from build123d import *

# Parameters (mm, degrees)
BOSS_EXTRUDE1_DEPTH = 3
SKETCH2_R           = 1.25
CUT_EXTRUDE1_DEPTH  = 16
CHAMFER1_SIZE       = 0.25
SKETCH3_R           = 4
CUT_EXTRUDE2_DEPTH  = 1
CUT_EXTRUDE3_DEPTH  = 11
CUT_EXTRUDE4_DEPTH  = 2
FILLET1_R           = 0.25
CUT_EXTRUDE5_DEPTH  = 3
SKETCH7_R           = 2.35
CUT_EXTRUDE6_DEPTH  = 3.5
CUT_EXTRUDE7_DEPTH  = 3.5
CIRPATTERN1_COUNT   = 24


with BuildPart() as part:
    # Sketch1 → Boss-Extrude1 (new body, symmetric)
    with BuildSketch(Plane(origin=(0, 0, 0), x_dir=(1, 0, 0), z_dir=(0, 1, 0))):
        with BuildLine():
            Line((23.75, 3.122009569), (9.501734608, 3.122009569))
            ThreePointArc((9.501734608, 3.122009569), (7.409369814, 3.580863286), (5.701040765, 4.873205742))
            ThreePointArc((5.701040765, 4.873205742), (-7.499303275, 0.102227183), (5.566088347, -5.026794258))
            ThreePointArc((5.566088347, -5.026794258), (7.246540637, -3.808746464), (9.276813911, -3.377990431))
            Line((9.276813911, -3.377990431), (23.75, -3.377990431))
            ThreePointArc((23.75, -3.377990431), (27, -0.127990431), (23.75, 3.122009569))
        make_face()
    extrude(amount=BOSS_EXTRUDE1_DEPTH, both=True)

    # Sketch2 → Cut-Extrude1 (cut)
    with BuildSketch(Plane(origin=(0, 3, 0), x_dir=(1, 0, 0), z_dir=(0, 1, 0))):
        with Locations((23.75, -0.127990431)):
            Circle(SKETCH2_R)
        with Locations((19.75, -0.127990431)):
            Circle(SKETCH2_R)
    extrude(amount=-CUT_EXTRUDE1_DEPTH, mode=Mode.SUBTRACT)

    # Chamfer1
    chamfer1_edges = [part.edges().sort_by_distance(p)[0] for p in [
        (22.5, 3, 0.127990431),
        (18.5, 3, 0.127990431),
    ]]
    chamfer(chamfer1_edges, length=CHAMFER1_SIZE)

    # Sketch3 → Cut-Extrude2 (cut)
    with BuildSketch(Plane(origin=(0, 3, 0), x_dir=(1, 0, 0), z_dir=(0, 1, 0))):
        Circle(SKETCH3_R)
    extrude(amount=-CUT_EXTRUDE2_DEPTH, mode=Mode.SUBTRACT)

    # Sketch4 → Cut-Extrude3 (cut)
    with BuildSketch(Plane(origin=(0, 3, 0), x_dir=(1, 0, 0), z_dir=(0, 1, 0))):
        with BuildLine():
            Line((-1.5, 1), (-9, 1))
            Line((-9, 1), (-9, -1))
            Line((-9, -1), (-1.5, -1))
            ThreePointArc((-1.5, -1), (-1.183772234, -1.051316702), (-0.9, -1.2))
            ThreePointArc((-0.9, -1.2), (0, -1.5), (0.9, -1.2))
            ThreePointArc((0.9, -1.2), (1.183772234, -1.051316702), (1.5, -1))
            Line((1.5, -1), (7.969223594, -1))
            ThreePointArc((7.969223594, -1), (8.204925854, -1.028174684), (8.427346441, -1.111111111))
            ThreePointArc((8.427346441, -1.111111111), (10.25, 0), (8.427346441, 1.111111111))
            ThreePointArc((8.427346441, 1.111111111), (8.204925854, 1.028174684), (7.969223594, 1))
            Line((7.969223594, 1), (1.5, 1))
            ThreePointArc((1.5, 1), (1.183772234, 1.051316702), (0.9, 1.2))
            ThreePointArc((0.9, 1.2), (0, 1.5), (-0.9, 1.2))
            ThreePointArc((-0.9, 1.2), (-1.183772234, 1.051316702), (-1.5, 1))
        make_face()
    extrude(amount=-CUT_EXTRUDE3_DEPTH, mode=Mode.SUBTRACT)

    # Sketch5 → Cut-Extrude4 (cut)
    with BuildSketch(Plane.XZ.offset(3)):
        with BuildLine():
            Line((24.055684797, -4.372009569), (19.49, -4.372009569))
            Line((19.49, -4.372009569), (6.737511188, -4.372009569))
            ThreePointArc((6.737511188, -4.372009569), (8.030233116, 0.154534121), (6.564314835, 4.627990431))
            Line((6.564314835, 4.627990431), (19.49, 4.627990431))
            Line((19.49, 4.627990431), (24.055684797, 4.627990431))
            ThreePointArc((24.055684797, 4.627990431), (27.230594245, 3.312899878), (28.545684797, 0.137990431))
            Line((28.545684797, 0.137990431), (28.545684797, 0.117990431))
            ThreePointArc((28.545684797, 0.117990431), (27.230594245, -3.056919017), (24.055684797, -4.372009569))
        make_face()
        with BuildLine():
            Line((24.055684797, 2.627990431), (19.49, 2.627990431))
            ThreePointArc((19.49, 2.627990431), (17.729304115, 1.898686316), (17, 0.137990431))
            Line((17, 0.137990431), (17, 0.117990431))
            ThreePointArc((17, 0.117990431), (17.729304115, -1.642705455), (19.49, -2.372009569))
            Line((19.49, -2.372009569), (24.055684797, -2.372009569))
            ThreePointArc((24.055684797, -2.372009569), (25.816380683, -1.642705455), (26.545684797, 0.117990431))
            Line((26.545684797, 0.117990431), (26.545684797, 0.137990431))
            ThreePointArc((26.545684797, 0.137990431), (25.816380683, 1.898686316), (24.055684797, 2.627990431))
        make_face(mode=Mode.SUBTRACT)
    extrude(amount=-CUT_EXTRUDE4_DEPTH, mode=Mode.SUBTRACT)

    # Fillet1
    fillet1_edges = [part.edges().sort_by_distance(p)[0] for p in [
        (25.816380683, -3, -1.642705455),
        (21.772842399, -3, -2.372009569),
        (17.729304115, -3, -1.642705455),
        (17, -3, 0.127990431),
        (17.729304115, -3, 1.898686316),
        (21.772842399, -3, 2.627990431),
        (25.816380683, -3, 1.898686316),
        (26.545684797, -3, 0.127990431),
    ]]
    fillet(fillet1_edges, radius=FILLET1_R)

    # Sketch6 → Cut-Extrude5 (cut)
    with BuildSketch(Plane.XZ.offset(1)):
        with BuildLine():
            Line((16.572326108, 2.507990431), (10.678705054, 2.507990431))
            Line((10.678705054, 2.507990431), (9.432782088, 2.507990431))
            ThreePointArc((9.432782088, 2.507990431), (10.490779488, -0.069105379), (8.754910472, -2.247990431))
            Line((8.754910472, -2.247990431), (10.678705054, -2.247990431))
            Line((10.678705054, -2.247990431), (16.572326108, -2.247990431))
            Line((16.572326108, -2.247990431), (18.365364688, -2.247990431))
            ThreePointArc((18.365364688, -2.247990431), (17.000002911, 0.131991595), (18.3722845, 2.507990431))
            Line((18.3722845, 2.507990431), (16.572326108, 2.507990431))
        make_face()
    extrude(amount=-CUT_EXTRUDE5_DEPTH, mode=Mode.SUBTRACT)

    # Sketch7 → Cut-Extrude6 (cut)
    with BuildSketch(Plane.XZ.offset(3)):
        Circle(SKETCH7_R)
    extrude(amount=-CUT_EXTRUDE6_DEPTH, mode=Mode.SUBTRACT)

    # Sketch8 → Cut-Extrude7 (cut)
    with BuildSketch(Plane.XZ.offset(3)):
        with BuildLine():
            ThreePointArc((-0.299151371, 2.330881476), (0, 2.35), (0.299151371, 2.330881476))
            Line((0.299151371, 2.330881476), (0, 2.84902685))
            Line((0, 2.84902685), (-0.299151371, 2.330881476))
        make_face()
    cut_extrude7 = extrude(amount=-CUT_EXTRUDE7_DEPTH, mode=Mode.SUBTRACT)

    # CirPattern1: Cut-Extrude7 ×24 about axis
    cirpattern1_axis = Axis((0, 0, 0), (0, 1, 0))
    for i in range(1, CIRPATTERN1_COUNT):
        add(cut_extrude7.rotate(cirpattern1_axis, i * 360 / CIRPATTERN1_COUNT), mode=Mode.SUBTRACT)


solid = part.part
Here's how the part is built. I have some questions about the finished solid (model axes, mm). A direction names the side the tool comes from. Coordinates: 2 decimals unless noted, no trailing zeros. Order: outer loops, then holes, each group sorted by start corner. A loop starts at its lowest first (then second) coordinate and runs counter-clockwise, first axis right, second up. Notation, with made-up numbers: M -30.5,1 L 17.5,1 A13 ccw 17.5,20 Z; hole C -12.75,56 d7. An arc over 180 degrees is marked long. Answer as CSV lines item,"result". Start each with the question number.
1. I want a section at D-D, the plane z = -6.25. Write out the boundary of the cut face in (x, y).
2. For pin 1 (1.5 mm diameter, centred on x = -0.5, z = -2, fed in from -Y); pin 2 (1.5 mm diameter, centred on x = 14.5, y = 1, fed in from +Z); pin 3 (3 mm diameter, centred on x = 5.5, y = 0.5, fed in from -Z); pin 4 (2.5 mm diameter, centred on x = 13, y = 1, fed in from -Z), each with a flat end and sliding along its axis, tell me the tip position at first contact or that it passes through.
3. I need wall thicknesses on line 1 (Z direction, x = 19.75, y = -1.3); line 2 (Z direction, x = 23.75, y = 1.5); line 3 (Z direction, x = 18, y = 0.55). Which ranges of each line are inside material? Lowest first, please. Write a range as [from, to].
4. I want a section at B-B, the plane x = 11.5. Write out the boundary of the cut face in (y, z), and give its area (3 significant figures).
5. On a 3-axis mill with a long thin cutter (end or side, diameter ignored), from which of +Z, -Z, +X, -X, +Y, -Y can I reach the whole of each face in a straight line? I mean faces 4 (the flat face through (22, -2, 2.628)), 5 (the cylindrical face through (0.1, 2.5, -4)), 6 (the flat face through (22, -2, -2.372)), 7 (the flat face through (14, 0, 2.508)). Say none if no direction works.
6. I want a section at A-A, the plane y = 1.25. Write out the boundary of the cut face in (x, z), and give its area (3 significant figures).
7. We'd pull the mould along X, two halves only. Please class faces 1 (the cylindrical face through (7.66, -2.01, -2.42)), 2 (the cylindrical face through (25.8, -1.89, -1.66)), 3 (the flat face through (0, -3, -4)): released by +X, released by -X, zero draft, split by the parting line, or undercut.
8. I want a section at C-C, the plane y = -1.35. Count the separate pieces of the cut face and the enclosed holes in it, and give its area (3 significant figures).
Recorded:
1,outline,"M -4.15,-3 L 4.15,-3 L 4.15,3 L -4.15,3 Z"
2,pin 1,"stops at y = -3"
2,pin 2,"stops at z = 3.38"
2,pin 3,"stops at z = -6.34"
2,pin 4,"stops at z = -3.12"
3,line 1,"z = [-2.37, -1.12], [1.38, 2.63]"
3,line 2,"z = [-3.12, -1.12], [1.38, 3.38]"
3,line 3,"z = [-3.12, -2.25], [-1.99, 2.25], [2.51, 3.38]"
4,outline,"M -1,-3.12 L 3,-3.12 L 3,3.38 L -1,3.38 L -1,2.51 L 2,2.51 L 2,-2.25 L -1,-2.25 Z"
4,area,"11.7 mm2"
5,face 4,"+Z, +X, -Y"
5,face 5,"+Y"
5,face 6,"-Z, +X, -Y"
5,face 7,"-Y"
6,outline,"M -7.43,-1 A7.5 ccw 5.7,-4.87 A5 cw 9.5,-3.12 L 23.75,-3.12 A3.25 ccw 23.75,3.38 L 9.28,3.38 A5 cw 5.57,5.03 A7.5 ccw -7.43,1 L -1.5,1 A1 ccw -0.9,1.2 A1.5 cw 0.9,1.2 A1 ccw 1.5,1 L 7.97,1 A1 ccw 8.43,1.11 A1.25 cw long 8.43,-1.11 A1 ccw 7.97,-1 L 1.5,-1 A1 ccw 0.9,-1.2 A1.5 cw -0.9,-1.2 A1 ccw -1.5,-1 Z; hole M 8.75,-2.25 L 18.37,-2.25 A2.75 cw 18.37,2.51 L 9.43,2.51 A2.75 cw Z; hole C 19.75,0.13 d2.5; hole C 23.75,0.13 d2.5"
6,area,"221 mm2"
7,face 1,"undercut"
7,face 2,"released by +X"
7,face 3,"zero draft"
8,separate pieces,"3"
8,enclosed holes,"2"
8,area,"172 mm2"
